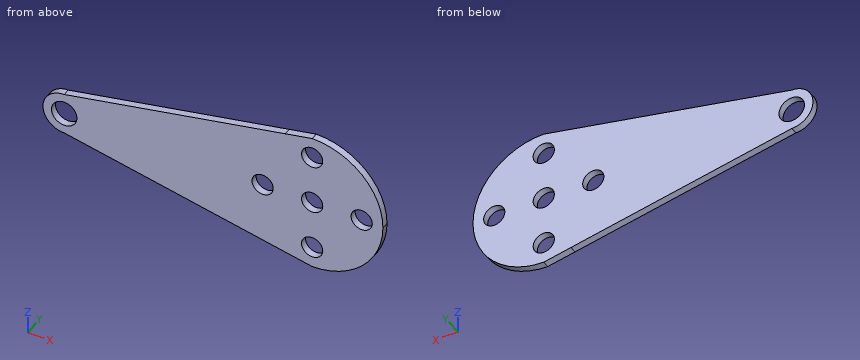
```python
from build123d import *

# Parameters (mm, degrees)
BOSS_EXTRUDE1_DEPTH = 1
SKETCH5_R           = 1.5
SKETCH5_R_2         = 1.8
CUT_EXTRUDE4_DEPTH  = 11


with BuildPart() as part:
    # Sketch1 → Boss-Extrude1 (new body)
    with BuildSketch(Plane(origin=(0, 0, 0), x_dir=(1, 0, 0), z_dir=(0, 1, 0))):
        with BuildLine():
            Line((0.003114812, 10.031035213), (0.003114812, 0.031035213))
            Line((0.003114812, 0.031035213), (0.003114812, -9.968964787))
            ThreePointArc((0.003114812, -9.968964787), (7.074182624, -7.040032599), (10.003114812, 0.031035213))
            ThreePointArc((10.003114812, 0.031035213), (7.074182624, 7.102103025), (0.003114812, 10.031035213))
        make_face()
        with BuildLine():
            Line((-32.050001176, 0.002656129), (-9.996881269, 0.022181449))
            ThreePointArc((-9.996881269, 0.022181449), (-8.322945106, 5.569692653), (-3.853372565, 9.257492015))
            Line((-3.853372565, 9.257492015), (-35.05, 3))
            ThreePointArc((-35.05, 3), (-32.929618948, 2.122259219), (-32.050001176, 0.002656129))
        make_face()
        with BuildLine():
            Line((-9.996881269, 0.022181449), (0.003114812, 0.031035213))
            Line((0.003114812, 0.031035213), (0.003114812, 10.031035213))
            Line((0.003114812, 10.031035213), (-3.853372565, 9.257492015))
            ThreePointArc((-3.853372565, 9.257492015), (-8.322945106, 5.569692653), (-9.996881269, 0.022181449))
        make_face()
        with BuildLine():
            Line((0.003114812, -9.968964787), (0.003114812, 0.031035213))
            Line((0.003114812, 0.031035213), (-9.996881269, 0.022181449))
            ThreePointArc((-9.996881269, 0.022181449), (-8.308581959, -5.529153344), (-3.821927798, -9.20850206))
            Line((-3.821927798, -9.20850206), (0.003114812, -9.968964787))
        make_face()
        with BuildLine():
            ThreePointArc((-3.821927798, -9.20850206), (-8.308581959, -5.529153344), (-9.996881269, 0.022181449))
            Line((-9.996881269, 0.022181449), (-32.050001176, 0.002656129))
            ThreePointArc((-32.050001176, 0.002656129), (-32.050000294, 0.001328065), (-32.05, 0))
            ThreePointArc((-32.05, 0), (-32.928679656, -2.121320344), (-35.05, -3))
            Line((-35.05, -3), (-3.821927798, -9.20850206))
        make_face()
        with BuildLine():
            ThreePointArc((-32.05, 0), (-32.050000294, 0.001328065), (-32.050001176, 0.002656129))
            Line((-32.050001176, 0.002656129), (-35.05, 0))
            Line((-35.05, 0), (-35.05, -3))
            ThreePointArc((-35.05, -3), (-32.928679656, -2.121320344), (-32.05, 0))
        make_face()
        with BuildLine():
            Line((-35.05, 0), (-32.050001176, 0.002656129))
            ThreePointArc((-32.050001176, 0.002656129), (-32.929618948, 2.122259219), (-35.05, 3))
            Line((-35.05, 3), (-35.05, 0))
        make_face()
        with BuildLine():
            Line((-35.05, 0), (-35.05, 3))
            ThreePointArc((-35.05, 3), (-38.05, 0), (-35.05, -3))
            Line((-35.05, -3), (-35.05, 0))
        make_face()
    extrude(amount=BOSS_EXTRUDE1_DEPTH)

    # Sketch5 → Cut-Extrude4 (cut)
    with BuildSketch(Plane.XZ):
        with Locations(Location((0, 0, 0), (0, 0, 270))):
            Circle(SKETCH5_R)
        with Locations(Location((0, 7, 0), (0, 0, 270))):
            Circle(SKETCH5_R)
        with Locations(Location((-35.05, 0, 0), (0, 0, 270))):
            Circle(SKETCH5_R_2)
        with Locations(Location((-7, 0, 0), (0, 0, 270))):
            Circle(SKETCH5_R)
        with Locations(Location((7, 0, 0), (0, 0, 270))):
            Circle(SKETCH5_R)
        with Locations(Location((0, -7, 0), (0, 0, 270))):
            Circle(SKETCH5_R)
    extrude(amount=-CUT_EXTRUDE4_DEPTH, mode=Mode.SUBTRACT)


solid = part.part
```
Build history of the part. All positions in model axes, mm. Give positions to 0.01 mm unless a question says otherwise; leave off trailing zeros. Loops run counter-clockwise (first coordinate to the right, second up) from the corner with the lowest first, then second, coordinate; pieces in that order, holes last. Notation, with made-up numbers: (-26.75, -29.75) - (-2.75, -29.75) arc R25 ccw to (-2.75, 7.25) - close; hole circle Ø9 at (0, 46). An arc over 180 degrees is marked (long way). Use a Markdown table: item, result.
(1) Band-saw the part on A-A (y = 0.4). Give the cut face in (x, z).
Taken from the geometry:
| item | result |
|---|---|
| outline | (-35.05, -3) - (0, -10.03) arc R10 ccw to (0, 9.97) - (-35.05, 3) arc R3 ccw to start; hole circle Ø3.6 at (-35.05, 0); hole circle Ø3 at (-7, 0); hole circle Ø3 at (0, -7); hole circle Ø3 at (0, 0); hole circle Ø3 at (0, 7); hole circle Ø3 at (7, 0) |
(2) Band-saw the part on D-D (x = 4.5). Give the cut face in (y, z), and give its area (3 significant figures).
Taken from the geometry:
| item | result |
|---|---|
| outline | (0, -8.96) - (1, -8.96) - (1, 8.9) - (0, 8.9) - close |
| area | 17.9 mm2 |
(3) Band-saw the part on C-C (z = -6). Give the cut face in (x, y), and give its area (3 significant figures).
Taken from the geometry:
| item | result |
|---|---|
| outline | (-20.09, 0) - (-1.12, 0) - (-1.12, 1) - (-20.09, 1) - close; (1.12, 0) - (8.03, 0) - (8.03, 1) - (1.12, 1) - close |
| area | 25.9 mm2 |
(4) Drop a flat-ended pin along its axis: pin 1 Ø2.5 at (x, z) = (7, 0) entering from +Y. Give the stop position or say it passes through.
Taken from the geometry:
| item | result |
|---|---|
| pin 1 | through |
(5) Wall check: line 1 along X through (y, z) = (0.3, 0); line 2 along X through (y, z) = (0.95, 0.5); line 3 along Z through (x, y) = (-10, 0.2). Give the ranges that are in metal, low to high.
Taken from the geometry:
| item | result |
|---|---|
| line 1 | -38.05 to -36.85, -33.25 to -8.5, -5.5 to -1.5, 1.5 to 5.5, 8.5 to 10 |
| line 2 | -38.01 to -36.78, -33.32 to -8.41, -5.59 to -1.41, 1.41 to 5.59, 8.41 to 9.99 |
| line 3 | -8.02 to 7.98 |
(6) Band-saw the part on B-B (x = -7). Give the cut face in (y, z).
Taken from the geometry:
| item | result |
|---|---|
| outline | (0, -8.63) - (1, -8.63) - (1, -1.5) - (0, -1.5) - close; (0, 1.5) - (1, 1.5) - (1, 8.58) - (0, 8.58) - close |
